from build123d import *

# Parameters (mm, degrees)
SKETCH_1_W          = 34.5
SKETCH_1_H          = 34.5
EXTRUDE_1_DEPTH     = 13.5
SKETCH_2_W          = 32.5
SKETCH_2_H          = 32.5
CUT_EXTRUDE_1_DEPTH = 2
SKETCH_3_W          = 30.5
SKETCH_3_H          = 30.5
CUT_EXTRUDE_2_DEPTH = 10
SKETCH_4_R          = 1.055259324
SKETCH_4_R_2        = 2.6
CUT_EXTRUDE_3_DEPTH = 12
CUT_EXTRUDE_4_REACH = 52.624
SKETCH_5_W          = 15.85
SKETCH_5_H          = 2.015973822
SKETCH_7_W          = 16.65
SKETCH_7_H          = 1
CUT_EXTRUDE_6_DEPTH = 10
SKETCH_8_W          = 9.5
SKETCH_8_H          = 1
CUT_EXTRUDE_7_DEPTH = 10


with BuildPart() as part:
    # 草图1 → 凸台-拉伸1 (new body)
    with BuildSketch(Plane(origin=(0, 0, 0), x_dir=(1, 0, 0), z_dir=(0, 1, 0))):
        with Locations((17.25, 17.25)):
            Rectangle(SKETCH_1_W, SKETCH_1_H)
    extrude(amount=EXTRUDE_1_DEPTH)

    # 草图2 → 切除-拉伸1 (cut)
    with BuildSketch(Plane(origin=(0, 13.5, 0), x_dir=(1, 0, 0), z_dir=(0, 1, 0))):
        with Locations((17.25, 17.25)):
            Rectangle(SKETCH_2_W, SKETCH_2_H)
    extrude(amount=-CUT_EXTRUDE_1_DEPTH, mode=Mode.SUBTRACT)

    # 草图3 → 切除-拉伸2 (cut)
    with BuildSketch(Plane(origin=(0, 11.5, 0), x_dir=(1, 0, 0), z_dir=(0, 1, 0))):
        with Locations((17.25, 17.25)):
            Rectangle(SKETCH_3_W, SKETCH_3_H)
    extrude(amount=-CUT_EXTRUDE_2_DEPTH, mode=Mode.SUBTRACT)

    # 草图4 → 切除-拉伸3 (cut)
    with BuildSketch(Plane(origin=(0, 1.5, 0), x_dir=(1, 0, 0), z_dir=(0, 1, 0))):
        with Locations(Location((3.25, 31.25, 0), (0, 0, 270))):
            Circle(SKETCH_4_R)
        with Locations(Location((31.25, 31.25, 0), (0, 0, 90))):
            Circle(SKETCH_4_R)
        with Locations(Location((31.25, 3.25, 0), (0, 0, 270))):
            Circle(SKETCH_4_R)
        with Locations(Location((3.25, 3.25, 0), (0, 0, 90))):
            Circle(SKETCH_4_R)
        with Locations(Location((17.25, 24.75, 0), (0, 0, 270))):
            Circle(SKETCH_4_R_2)
        with Locations(Location((17.25, 9.75, 0), (0, 0, 90))):
            Circle(SKETCH_4_R_2)
    extrude(amount=-CUT_EXTRUDE_3_DEPTH, mode=Mode.SUBTRACT)

    # 切除-拉伸4: up to this face of the body (flat: up to its plane)
    cut_extrude_4_end = Plane(part.part.faces().sort_by_distance((17.25, 1.5, -17.25))[0])
    # 草图5 → 切除-拉伸4 (cut, up to the picked face)
    with BuildSketch(Plane(origin=(0, 13.5, 0), x_dir=(1, 0, 0), z_dir=(0, 1, 0)), mode=Mode.PRIVATE) as cut_extrude_4_sk1:
        with Locations((25.575, 33.492013089)):
            Rectangle(SKETCH_5_W, SKETCH_5_H)
    cut_extrude_4_tool1 = split(extrude(cut_extrude_4_sk1.sketch, amount=-CUT_EXTRUDE_4_REACH, mode=Mode.PRIVATE), bisect_by=cut_extrude_4_end, keep=Keep.BOTH, mode=Mode.PRIVATE)
    add(cut_extrude_4_tool1.solids().sort_by(Axis((25.575, 13.5, -33.492013), (0, -1, 0)))[0], mode=Mode.SUBTRACT)

    # 草图7 → 切除-拉伸6 (cut)
    with BuildSketch(Plane(origin=(0, 11.5, 0), x_dir=(1, 0, 0), z_dir=(0, 1, 0))):
        with Locations((9.325, 33)):
            Rectangle(SKETCH_7_W, SKETCH_7_H)
    extrude(amount=-CUT_EXTRUDE_6_DEPTH, mode=Mode.SUBTRACT)

    # 草图8 → 切除-拉伸7 (cut)
    with BuildSketch(Plane(origin=(0, 11.5, 0), x_dir=(1, 0, 0), z_dir=(0, 1, 0))):
        with Locations((9.75, 1.5)):
            Rectangle(SKETCH_8_W, SKETCH_8_H)
    extrude(amount=-CUT_EXTRUDE_7_DEPTH, mode=Mode.SUBTRACT)


solid = part.part
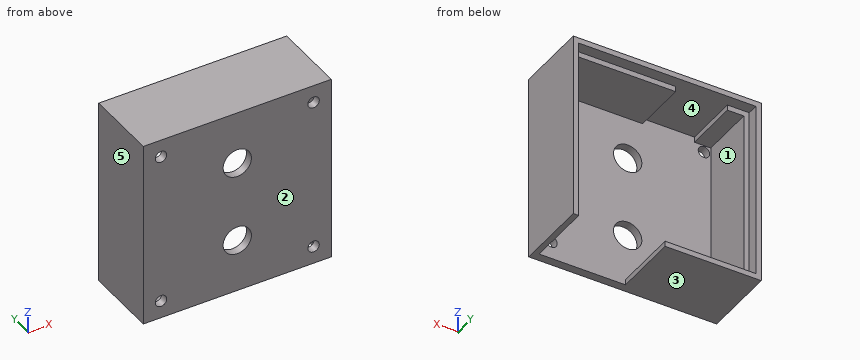
Input: part model. Units: mm. Frame: model coordinates. Face numbers are marked on the shaded views. A direction names the side the tool comes from. Coordinates: 2 decimals unless noted, no trailing zeros. Write each loop counter-clockwise with the first axis right and the second up, starting at its lowest first coordinate (ties: lowest second). Pieces come first, ordered by that corner, then holes. Notation, with made-up numbers: M -6,59 L 46,59 A20 cw 46,75 Z; hole C 59.25,-23 d4. An arc over 180 degrees is marked long. Answer as a JSON object with one key per item and string values. Group by question number.
(1) Mould query, pull axis X, two halves, no side actions, for the marked faces 3, 4 and 5. Classes: pulls with the +X half, pulls with the -X half, needs draft (parallel to the pull), parting line crosses it, or undercut.
(2) Contact query for a flat-ended pin moving along its axis: P1, Ø1, axis at x = 6.5, z = -27.5, coming from the +Y side. Output: stop coordinate, or through.
(3) Section B-B on z = -31.25. Output: boundary loops of the cut face in (x, y).
(4) Set-up query: the marked faces 1 and 2. Return all of +Z, -Z, +X, -X, +Y, -Y with unobstructed straight access to the full face (end or side cutting, diameter ignored); none if empty.
(5) Ray query, line 1 along X through (y, z) = (0.9, -3.25); line 2 along X through (y, z) = (0.95, -24.75); line 3 along X through (y, z) = (8.5, -9). Return the intervals inside material, ascending. Write a range as [from, to].
(6) Section D-D on x = 23.5. Output: boundary loops of the cut face in (y, z).
(7) Section C-C on x = 31.25. Output: boundary loops of the cut face in (y, z), plus the area to 3 significant figures.
(8) Section A-A on z = -24.75. Output: boundary loops of the cut face in (x, y).
Result set:
{
 "1": {"face 3": "needs draft", "face 4": "undercut", "face 5": "pulls with the -X half"},
 "2": {"P1": "stops at y = 1.5"},
 "3": {"outline": "M 0,0 L 2.19,0 L 2.19,1.5 L 2,1.5 L 2,11.5 L 1,11.5 L 1,13.5 L 0,13.5 Z; M 4.31,0 L 30.19,0 L 30.19,1.5 L 4.31,1.5 Z; M 32.31,0 L 34.5,0 L 34.5,13.5 L 33.5,13.5 L 33.5,11.5 L 32.5,11.5 L 32.5,1.5 L 32.31,1.5 Z"},
 "4": {"face 1": "+Y", "face 2": "+Z, -Z, +X, -X, -Y"},
 "5": {"line 1": "x = [0, 2.19], [4.31, 30.19], [32.31, 34.5]", "line 2": "x = [0, 14.65], [19.85, 34.5]", "line 3": "x = [0, 2], [32.5, 34.5]"},
 "6": {"outline": "M 0,-34.5 L 1.5,-34.5 L 1.5,-2 L 11.5,-2 L 11.5,-1 L 13.5,-1 L 13.5,0 L 0,0 Z"},
 "7": {"outline": "M 0,-34.5 L 1.5,-34.5 L 1.5,-32.31 L 0,-32.31 Z; M 0,-30.19 L 1.5,-30.19 L 1.5,-4.31 L 0,-4.31 Z; M 0,-2.19 L 1.5,-2.19 L 1.5,-2 L 11.5,-2 L 11.5,-1 L 13.5,-1 L 13.5,0 L 0,0 Z", "area": "67.4 mm2"},
 "8": {"outline": "M 0,0 L 14.65,0 L 14.65,1.5 L 2,1.5 L 2,11.5 L 1,11.5 L 1,13.5 L 0,13.5 Z; M 19.85,0 L 34.5,0 L 34.5,13.5 L 33.5,13.5 L 33.5,11.5 L 32.5,11.5 L 32.5,1.5 L 19.85,1.5 Z"}
}
